Build history of the part. All positions in model axes, mm. Give positions to 0.01 mm unless a question says otherwise; leave off trailing zeros. Order: outer loops, then holes, each group sorted by start corner. A loop starts at its lowest first (then second) coordinate and runs counter-clockwise, first axis right, second up. Notation, with made-up numbers: (-38.75, -19.5) - (-14.75, -19.5) arc R22 cw to (-14.75, 9.5) - close; hole circle Ø8 at (66.25, 2.25). An arc over 180 degrees is marked (long way). Use a Markdown table: item, result. Add a question column.
(1) Wall check: line 1 (X direction, y = 0.8, z = 0); line 2 (Y direction, x = 4.5, z = 17). Give the ranges that are in metal, low to high.
(2) Slice it at B-B (y = 3.5). Count the separate pieces of the cut face and the enclosed holes in it, then the cut area to 3 significant figures.
(3) Flat gauge pins, fed straight in: pin 1 (1 mm diameter, centred on y = 2, z = -1, fed in from +X); pin 2 (2 mm diameter, centred on y = 6.5, z = 18, fed in from +X); pin 3 (1.5 mm diameter, centred on y = 8, z = 8.5, fed in from +X). Where does each tip first touch, or does it go through?
(4) Slice it at A-A (y = 10.25). Write the cut outline in (x, z) (1 decimal).
(5) Mould opens along Z. For faces 1 (the face through (-23.754, 3.764, 11.137)), 2 (the face through (26.033, 3.704, 3.252)) say: +Z half, -Z half, draft (parallel to the pull), parting line (faces both ways), or undercut.
from build123d import *

# Parameters (mm, degrees)
SKETCH2_R               = 26.9875
BOSS_EXTRUDE1_DEPTH     = 11.5951
SHELL1_T                = -1.5875
CUT_EXTRUDE1_DEPTH      = 40.456334983
CUT_EXTRUDE1_DEPTH_BACK = 40.456334983
SKETCH5_R               = 12.7
CUT_EXTRUDE2_DEPTH      = 38.1
CIRPATTERN3_COUNT       = 20


with BuildPart() as part:
    # Sketch2 → Boss-Extrude1 (new body)
    with BuildSketch(Plane(origin=(0, 0, 0), x_dir=(1, 0, 0), z_dir=(0, 1, 0))):
        with Locations(Location((0, 0, 0), (0, 0, 270))):
            Circle(SKETCH2_R)
    extrude(amount=BOSS_EXTRUDE1_DEPTH)

    # Shell1
    shell1_openings = [part.faces().sort_by_distance(p)[0] for p in [
        (0, 11.5951, 0),
    ]]
    offset(amount=SHELL1_T, openings=shell1_openings, kind=Kind.INTERSECTION)

    # Sketch5 → Cut-Extrude1 (cut, two sides: drawn at the far end of the back side and taken through both)
    with BuildSketch(Plane(origin=(0, 1.5875, 0), x_dir=(1, 0, 0), z_dir=(0, 1, 0)).offset(-CUT_EXTRUDE1_DEPTH_BACK)):
        with Locations(Location((0, 0, 0), (0, 0, 270))):
            Circle(SKETCH5_R)
    extrude(amount=CUT_EXTRUDE1_DEPTH + CUT_EXTRUDE1_DEPTH_BACK, mode=Mode.SUBTRACT)

    # Sketch6 → Cut-Extrude2 (cut)
    with BuildSketch(Plane.XY):
        Polygon((0, 1.5875), (6.413577678, 1.5875), (0, 5.8801), (-6.413577678, 5.8801), align=None)
    cut_extrude2 = extrude(amount=-CUT_EXTRUDE2_DEPTH, mode=Mode.SUBTRACT)

    # CirPattern3: Cut-Extrude2 ×20 about axis
    cirpattern3_axis = Axis((0, 0, 0), (0, 1, 0))
    for i in range(1, CIRPATTERN3_COUNT):
        add(cut_extrude2.rotate(cirpattern3_axis, i * 360 / CIRPATTERN3_COUNT), mode=Mode.SUBTRACT)


solid = part.part
Solution:
| question | item | result |
|---|---|---|
| 1 | line 1 | -26.99 to -12.7, 12.7 to 26.99 |
| 1 | line 2 | 0 to 1.59 |
| 2 | separate pieces | 20 |
| 2 | enclosed holes | 0 |
| 2 | area | 57.1 mm2 |
| 3 | pin 1 | x = 26.98 |
| 3 | pin 2 | x = 20.96 |
| 3 | pin 3 | x = 25.85 |
| 4 | outline | circle Ø54 at (0, 0); hole circle Ø50.8 at (0, 0) |
| 5 | face 1 | undercut |
| 5 | face 2 | undercut |
